Geometry: final body of the model. Coordinates: model frame, mm. A direction names the side the tool comes from. Give positions to 0.01 mm unless a question says otherwise; leave off trailing zeros. Loops run counter-clockwise (first coordinate to the right, second up) from the corner with the lowest first, then second, coordinate; pieces in that order, holes last. Notation, with made-up numbers: (7, 83) -> (35, 83) arc R22 cw to (35, 91) -> close; hole circle Ø1 at (62.25, -4.5). An arc over 180 degrees is marked (long way). Answer in a Markdown table with one row per item. Add a question column.
1) Section query A-A (z = 55). Return the cut outline in (x, y), plus the area to 3 significant figures.
2) Access query for faces 1 (the flat face through (54, 16, 32.004)), 2 (the flat face through (57, 38.1, 30)), 3 (the flat face through (21.59, 57, 35)), 4 (the flat face through (38.1, 35, 19)), 5 (the flat face through (35, 19, 38.1)). Directions: +Z, -Z, +X, -X, +Y, -Y. A direction counts if a zero-diameter tool reaches every point of the face in a straight line with its end or side. Return the directions, or none.
3) First-contact query: P1, Ø1.5, axis at y = 36, z = 20, coming from the +X side; P2, Ø4, axis at x = 34, y = 19.5, coming from the +Z side; P3, Ø1, axis at x = 44, z = 9, coming from the +Y side. Flat tips, straight axial feed; report the tip coordinate or a pass-through.
4) Line query: line 1 (Y direction, x = 52, z = 24); line 2 (Y direction, x = 38, z = 63). Output: solid intervals per line, ascending. Write a range as from..to.
5) Section query C-C (x = 34.5). Return the cut outline in (y, z), plus the area to 3 significant figures.
6) Draft query along X for faces 6 (the flat face through (0, 29, 29)), 7 (the flat face through (29, 29, 0)), 8 (the flat face through (33, 6.35, 26)). Return one class per face: +X half, -X half, draft (parallel to the pull), parting line (faces both ways), or undercut.
Autodesk Inventor part; units mm, degrees
ref_plane "YZ Plane" through (0, 0, 0) normal (1, 0, 0) x (0, 1, 0)
ref_plane "XZ Plane" through (0, 0, 0) normal (0, 1, 0) x (-1, 0, 0)
ref_plane "XY Plane" through (0, 0, 0) normal (0, 0, 1) x (1, 0, 0)
sketch "Sketch1" plane through (0, 0, 0) normal (0, 0, 1) x (1, 0, 0)
  line L0 (0, 0) -> (38.1, 0)
  line L1 (38.1, 0) -> (38.1, 38.1)
  line L2 (38.1, 38.1) -> (0, 38.1)
  line L3 (0, 38.1) -> (0, 0)
  dimension "d0" = 38.1
  dimension "d1" = 38.1
extrude "Extrusion1" add sketch "Sketch1" along normal blind 38.1
sketch "Sketch2" plane through (0, 0, 38.1) normal (0, 0, 1) x (1, 0, 0)
  line L0 (6.35, 6.35) -> (32.004, 6.35)
  line L1 (32.004, 6.35) -> (32.004, 32.004)
  line L2 (32.004, 32.004) -> (6.35, 32.004)
  line L3 (6.35, 32.004) -> (6.35, 6.35)
  line L4 (38.1, 0) -> (38.1, 38.1)
  line L5 (0, 0) -> (38.1, 0)
  line L6 (38.1, 0) -> (38.1, 38.1)
  line L7 (38.1, 38.1) -> (0, 38.1)
  line L8 (0, 38.1) -> (0, 0)
  dimension "d4" = 25.654
  dimension "d5" = 25.654
extrude "Extrusion2" cut sketch "Sketch2" against normal blind 31.75 contours L3 L2 L1 L0
sketch "Sketch3" plane through (38.1, 0, 0) normal (1, 0, 0) x (0, 0, -1)
  point P0 (0, 0)
sketch "Sketch5" plane through (0, 0, 38.1) normal (0, 0, 1) x (1, 0, 0)
  line L0 (6.35, 6.35) -> (6.35, 32.004)
  line L1 (6.35, 6.35) -> (32.004, 6.35)
  line L2 (32.004, 6.35) -> (32.004, 32.004)
  line L3 (32.004, 32.004) -> (6.35, 32.004)
  line L4 (6.35, 32.004) -> (6.35, 6.35)
  line L5 (0, 0) -> (38.1, 0)
  line L6 (0, 0) -> (38.1, 0)
  line L7 (38.1, 0) -> (38.1, 38.1)
  line L8 (38.1, 38.1) -> (0, 38.1)
  line L9 (0, 38.1) -> (0, 0)
extrude "Extrusion4" add sketch "Sketch5" along normal blind 38.1
sketch "Sketch7" plane through (38.1, 0, 0) normal (1, 0, 0) x (0, 0, -1)
  line L0 (0, 0) -> (-76.2, 0)
  line L1 (0, 0) -> (-38.1, 0)
  line L2 (-38.1, 0) -> (-38.1, 38.1)
  line L3 (-38.1, 38.1) -> (0, 38.1)
  line L4 (0, 38.1) -> (0, 0)
  line L5 (-76.2, 6.35) -> (-6.35, 6.35)
  line L6 (-6.35, 6.35) -> (-32.004, 6.35)
  line L7 (-32.004, 6.35) -> (-32.004, 32.004)
  line L8 (-32.004, 32.004) -> (-6.35, 32.004)
  line L9 (-6.35, 32.004) -> (-6.35, 6.35)
  dimension "d16" = 38.1
  dimension "d17" = 38.1
  dimension "d20" = 25.654
  dimension "d21" = 25.654
extrude "Extrusion6" add sketch "Sketch7" along normal blind 38.1
sketch "Sketch9" plane through (38.1, 6.35, 6.35) normal (1, 0, 0) x (0, 0, -1)
  line L0 (-25.654, 0) -> (-25.654, 25.654)
  line L1 (0, 0) -> (0, 25.654)
  line L2 (-25.654, 0) -> (0, 0)
  line L3 (0, 0) -> (0, 25.654)
  line L4 (0, 25.654) -> (-25.654, 25.654)
  line L5 (-25.654, 25.654) -> (-25.654, 0)
  point P0 (6.35, -6.35)
extrude "Extrusion7" cut sketch "Sketch9" against normal blind 31.75
sketch "Sketch10" plane through (0, 38.1, 76.2) normal (0, 1, 0) x (1, 0, 0)
  line L0 (76.2, 69.85) -> (6.35, 69.85)
  line L1 (6.35, 69.85) -> (32.004, 69.85)
  line L2 (32.004, 69.85) -> (32.004, 44.196)
  line L3 (32.004, 44.196) -> (6.35, 44.196)
  line L4 (6.35, 44.196) -> (6.35, 69.85)
  line L5 (38.1, 38.1) -> (38.1, 0)
  line L6 (0, 76.2) -> (0, 0)
  line L7 (38.1, 38.1) -> (0, 38.1)
  line L8 (0, 38.1) -> (0, 76.2)
  line L9 (0, 76.2) -> (38.1, 76.2)
  line L10 (38.1, 76.2) -> (38.1, 38.1)
  point P0 (0, 38.1)
  dimension "d26" = 25.654
  dimension "d27" = 25.654
extrude "Extrusion8" add sketch "Sketch10" along normal blind 38.1
sketch "Sketch11" plane through (6.35, 38.1, 6.35) normal (0, 1, 0) x (1, 0, 0)
  line L0 (0, -25.654) -> (25.654, -25.654)
  line L1 (25.654, -25.654) -> (0, -25.654)
  line L2 (0, -25.654) -> (0, 0)
  line L3 (0, 0) -> (25.654, 0)
  line L4 (25.654, 0) -> (25.654, -25.654)
  point P0 (-6.35, 6.35)
extrude "Extrusion9" cut sketch "Sketch11" against normal blind 6.35
sketch "Sketch12" plane through (0, 76.2, 76.2) normal (0, 1, 0) x (1, 0, 0)
  line L0 (38.1, 55.88) -> (32.004, 55.88)
  line L1 (32.004, 55.88) -> (32.004, 58.42)
  line L2 (32.004, 58.42) -> (38.1, 58.42)
  line L3 (38.1, 58.42) -> (38.1, 55.88)
  point P0 (0, 76.2)
  dimension "d32" = 6.096
  dimension "d33" = 2.54
extrude "Extrusion10" cut sketch "Sketch12" against normal blind 38.1
sketch "Sketch13" plane through (76.2, 38.1, 38.1) normal (0, 1, 0) x (1, 0, 0)
  line L0 (0, 31.75) -> (0, 6.096)
  line L1 (-44.196, 17.78) -> (0, 17.78)
  line L2 (0, 17.78) -> (0, 20.32)
  line L3 (0, 20.32) -> (-44.196, 20.32)
  line L4 (-44.196, 20.32) -> (-44.196, 17.78)
  point P0 (-76.2, 38.1)
  dimension "d36" = 2.54
extrude "Extrusion11" cut sketch "Sketch13" against normal blind 6.35
sketch "Sketch15" plane through (0, 76.2, 76.2) normal (0, 1, 0) x (1, 0, 0)
  line L0 (17.78, 38.1) -> (20.32, 38.1)
  line L1 (20.32, 38.1) -> (20.32, 44.196)
  line L2 (20.32, 44.196) -> (17.78, 44.196)
  line L3 (17.78, 44.196) -> (17.78, 38.1)
  point P0 (0, 76.2)
  dimension "d39" = 2.54
  dimension "d40" = 6.096
extrude "Extrusion12" cut sketch "Sketch15" against normal blind 38.1
sketch "Sketch16" plane through (0, 38.1, 76.2) normal (0, 1, 0) x (1, 0, 0)
  line L0 (20.32, 44.196) -> (20.32, 38.1)
  line L1 (0, 0) -> (38.1, 0)
  line L2 (20.32, 44.196) -> (17.78, 44.196)
  line L3 (17.78, 44.196) -> (17.78, 0)
  line L4 (17.78, 0) -> (20.32, 0)
  line L5 (20.32, 0) -> (20.32, 44.196)
  point P0 (0, 76.2)
  dimension "d43" = 2.54
extrude "Extrusion13" cut sketch "Sketch16" against normal blind 6.35
sketch "Sketch17" plane through (38.1, 0, 76.2) normal (1, 0, 0) x (0, 0, -1)
  line L0 (38.1, 0) -> (38.1, 38.1)
  line L1 (0, 17.78) -> (38.1, 17.78)
  line L2 (38.1, 17.78) -> (38.1, 20.32)
  line L3 (38.1, 20.32) -> (0, 20.32)
  line L4 (0, 20.32) -> (0, 17.78)
  point P0 (76.2, 0)
  dimension "d46" = 2.54
extrude "Extrusion14" cut sketch "Sketch17" against normal blind 6.35
sketch "Sketch18" plane through (38.1, 0, 38.1) normal (0, 0, 1) x (1, 0, 0)
  line L0 (0, 17.78) -> (38.1, 17.78)
  line L1 (38.1, 17.78) -> (38.1, 20.32)
  line L2 (38.1, 20.32) -> (0, 20.32)
  line L3 (0, 20.32) -> (0, 17.78)
  point P0 (-38.1, 0)
  dimension "d49" = 38.1
  dimension "d50" = 2.54
extrude "Extrusion15" cut sketch "Sketch18" against normal blind 6.35
sketch "Sketch20" plane through (38.1, 38.1, 38.1) normal (0, 0, 1) x (1, 0, 0)
  line L0 (-17.78, -6.096) -> (-17.78, 38.1)
  line L1 (0, 0) -> (-17.78, 0)
  line L2 (-17.78, 38.1) -> (-16.51, 38.1)
  line L3 (-16.51, 38.1) -> (-16.51, 0)
  line L4 (-16.51, 0) -> (-17.78, 0)
  line L5 (-17.78, 0) -> (-17.78, 38.1)
  point P0 (-38.1, -38.1)
  dimension "d53" = 1.27
extrude "Extrusion16" cut sketch "Sketch20" against normal blind 6.35
sketch "Sketch21" plane through (38.1, 38.1, 76.2) normal (0, 1, 0) x (1, 0, 0)
  line L0 (-17.78, 0) -> (-17.78, 44.196)
  line L1 (0, 0) -> (-17.78, 0)
  line L2 (-17.78, 44.196) -> (-16.51, 44.196)
  line L3 (-16.51, 44.196) -> (-16.51, 0)
  line L4 (-16.51, 0) -> (-17.78, 0)
  line L5 (-17.78, 0) -> (-17.78, 44.196)
  point P0 (-38.1, 76.2)
  dimension "d56" = 1.27
extrude "Extrusion17" cut sketch "Sketch21" against normal blind 6.35
sketch "Sketch23" plane through (0, 38.1, 38.1) normal (0, 0, 1) x (1, 0, 0)
  line L0 (17.78, 0) -> (17.78, 38.1)
  line L1 (17.78, 0) -> (0, 0)
  line L2 (17.78, 38.1) -> (16.51, 38.1)
  line L3 (16.51, 38.1) -> (16.51, 0)
  line L4 (16.51, 0) -> (17.78, 0)
  line L5 (17.78, 0) -> (17.78, 38.1)
  point P0 (0, -38.1)
  dimension "d59" = 1.27
extrude "Extrusion18" cut sketch "Sketch23" against normal blind 6.35
sketch "Sketch24" plane through (0, 38.1, 76.2) normal (0, 1, 0) x (1, 0, 0)
  line L0 (17.78, 44.196) -> (17.78, 0)
  line L1 (17.78, 0) -> (0, 0)
  line L2 (17.78, 44.196) -> (16.51, 44.196)
  line L3 (16.51, 44.196) -> (16.51, 0)
  line L4 (16.51, 0) -> (17.78, 0)
  line L5 (17.78, 0) -> (17.78, 44.196)
  point P0 (0, 76.2)
  dimension "d62" = 1.27
extrude "Extrusion19" cut sketch "Sketch24" against normal blind 6.35
sketch "Sketch25" plane through (38.1, 0, 76.2) normal (1, 0, 0) x (0, 0, -1)
  line L0 (38.1, 0) -> (38.1, 17.78)
  line L1 (38.1, 17.78) -> (0, 17.78)
  line L2 (0, 17.78) -> (0, 16.51)
  line L3 (0, 16.51) -> (38.1, 16.51)
  line L4 (38.1, 16.51) -> (38.1, 17.78)
  point P0 (76.2, 0)
  dimension "d65" = 38.1
  dimension "d66" = 1.27
extrude "Extrusion20" cut sketch "Sketch25" against normal blind 6.35
sketch "Sketch26" plane through (38.1, 38.1, 76.2) normal (1, 0, 0) x (0, 0, -1)
  line L0 (0, -17.78) -> (38.1, -17.78)
  line L1 (38.1, -17.78) -> (0, -17.78)
  line L2 (0, -17.78) -> (0, -16.51)
  line L3 (0, -16.51) -> (38.1, -16.51)
  line L4 (38.1, -16.51) -> (38.1, -17.78)
  point P0 (76.2, -38.1)
  dimension "d69" = 38.1
  dimension "d70" = 1.27
extrude "Extrusion21" cut sketch "Sketch26" against normal blind 6.35
sketch "Sketch27" plane through (38.1, 0, 38.1) normal (0, 0, 1) x (1, 0, 0)
  line L0 (0, 21.59) -> (0, 38.1)
  line L1 (0, 20.32) -> (38.1, 20.32)
  line L2 (0, 21.59) -> (38.1, 21.59)
  line L3 (38.1, 21.59) -> (38.1, 20.32)
  line L4 (38.1, 20.32) -> (0, 20.32)
  line L5 (0, 20.32) -> (0, 21.59)
  line L6 (38.1, 17.78) -> (0, 17.78)
  line L7 (0, 17.78) -> (38.1, 17.78)
  line L8 (38.1, 17.78) -> (38.1, 16.51)
  line L9 (38.1, 16.51) -> (0, 16.51)
  line L10 (0, 16.51) -> (0, 17.78)
  point P0 (-38.1, 0)
  dimension "d73" = 38.1
  dimension "d74" = 1.27
extrude "Extrusion22" cut sketch "Sketch27" against normal blind 6.35
sketch "Sketch28" plane through (38.1, 38.1, 38.1) normal (0, 1, 0) x (1, 0, 0)
  line L0 (0, 20.32) -> (38.1, 20.32)
  line L1 (0, 20.32) -> (38.1, 20.32)
  line L2 (38.1, 20.32) -> (38.1, 21.59)
  line L3 (38.1, 21.59) -> (0, 21.59)
  line L4 (0, 21.59) -> (0, 20.32)
  line L5 (-6.096, 17.78) -> (38.1, 17.78)
  line L6 (38.1, 17.78) -> (0, 17.78)
  line L7 (0, 17.78) -> (0, 16.51)
  line L8 (0, 16.51) -> (38.1, 16.51)
  line L9 (38.1, 16.51) -> (38.1, 17.78)
  point P0 (-38.1, 38.1)
  point P1 (0, 17.78)
  dimension "d77" = 38.1
  dimension "d78" = 1.27
  dimension "d79" = 38.1
  dimension "d80" = 1.27
extrude "Extrusion23" cut sketch "Sketch28" against normal blind 6.35
sketch "Sketch29" plane through (38.1, 38.1, 0) normal (1, 0, 0) x (0, 0, -1)
  line L0 (-17.78, -6.096) -> (-6.35, -6.096)
  line L1 (-6.35, 38.1) -> (-17.78, 38.1)
  line L2 (-17.78, -6.096) -> (-16.51, -6.096)
  line L3 (-16.51, -6.096) -> (-16.51, 38.1)
  line L4 (-16.51, 38.1) -> (-17.78, 38.1)
  line L5 (-17.78, 38.1) -> (-17.78, -6.096)
  line L6 (-21.59, 0) -> (-21.59, -6.096)
  line L7 (-20.32, 38.1) -> (-20.32, -6.096)
  line L8 (-21.59, -6.096) -> (-20.32, -6.096)
  line L9 (-20.32, -6.096) -> (-20.32, 38.1)
  line L10 (-20.32, 38.1) -> (-21.59, 38.1)
  line L11 (-21.59, 38.1) -> (-21.59, -6.096)
  point P0 (0, -38.1)
  point P1 (-20.32, -6.096)
  dimension "d83" = 1.27
extrude "Extrusion24" cut sketch "Sketch29" against normal blind 6.35
sketch "Sketch30" plane through (76.2, 38.1, 21.59) normal (0, 0, -1) x (-1, 0, 0)
  line L0 (0, 0) -> (38.1, 0)
  line L1 (44.196, 38.1) -> (44.196, -6.096)
  line L2 (38.1, 0) -> (44.196, 0)
  line L3 (44.196, 0) -> (44.196, -6.096)
  line L4 (44.196, -6.096) -> (38.1, -6.096)
  line L5 (38.1, -6.096) -> (38.1, 0)
  point P0 (76.2, -38.1)
  point P1 (44.196, 0)
extrude "Extrusion25" add sketch "Sketch30" along normal blind 5.08
sketch "Sketch31" plane through (21.59, 38.1, 38.1) normal (-1, 0, 0) x (0, 0, 1)
  line L0 (38.1, -6.096) -> (-6.096, -6.096)
  line L1 (0, 0) -> (-6.096, 0)
  line L2 (-6.096, 0) -> (-6.096, -6.096)
  line L3 (-6.096, -6.096) -> (0, -6.096)
  line L4 (0, -6.096) -> (0, 0)
  point P0 (-38.1, -38.1)
extrude "Extrusion26" add sketch "Sketch31" along normal blind 5.08
properties part number "corner connector"
Evaluation:
| question | item | result |
|---|---|---|
| 1 | outline | (0, 0) -> (38.1, 0) -> (38.1, 16.51) -> (32, 16.51) -> (32, 6.35) -> (6.35, 6.35) -> (6.35, 32) -> (16.51, 32) -> (16.51, 38.1) -> (0, 38.1) -> close; (21.59, 32) -> (32, 32) -> (32, 21.59) -> (38.1, 21.59) -> (38.1, 38.1) -> (21.59, 38.1) -> close |
| 1 | area | 732 mm² |
| 2 | face 1 | +X |
| 2 | face 2 | +Z, -Z, +X, +Y |
| 2 | face 3 | +Z, +Y |
| 2 | face 4 | +X, +Y |
| 2 | face 5 | +Z, +X |
| 3 | P1 | x = 38.1 |
| 3 | P2 | z = 38.1 |
| 3 | P3 | y = 38.1 |
| 4 | line 1 | 0..6.35, 32..38.1 |
| 4 | line 2 | 0..16.51, 21.59..38.1 |
| 5 | outline | (0, 0) -> (76.2, 0) -> (76.2, 16.51) -> (38.1, 16.51) -> (38.1, 21.59) -> (76.2, 21.59) -> (76.2, 38.1) -> (38.1, 38.1) -> (38.1, 76.2) -> (21.59, 76.2) -> (21.59, 38.1) -> (16.51, 38.1) -> (16.51, 76.2) -> (0, 76.2) -> close; hole (6.35, 6.35) -> (32, 6.35) -> (32, 32) -> (6.35, 32) -> close |
| 5 | area | 3,310 mm² |
| 6 | face 6 | -X half |
| 6 | face 7 | draft |
| 6 | face 8 | undercut |
